from build123d import *

# Parameters (mm, degrees)
SKETCH1_R               = 27.75
SKETCH1_R_2             = 25.75
BOSS_EXTRUDE1_DEPTH     = 2.5
BOSS_EXTRUDE2_START     = -32.750000066
BOSS_EXTRUDE2_OUTLINE_R = 2.5
BOSS_EXTRUDE2_DEPTH     = 65.500000132
BOSS_EXTRUDE2_START_2   = -3
BOSS_EXTRUDE2_2_DEPTH   = 6
CUT_EXTRUDE1_DEPTH      = 43.998546635
CUT_EXTRUDE1_DEPTH_BACK = 43.998546635
SKETCH3_R               = 25.75


with BuildPart() as part:
    # Sketch1 → Boss-Extrude1 (new, symmetric)
    with BuildSketch(Plane(origin=(0, 0, 0), x_dir=(1, 0, 0), z_dir=(0, 1, 0))):
        with Locations(Location((0, 0, 0), (0, 0, 270))):
            Circle(SKETCH1_R)
        with Locations(Location((0, 0, 0), (0, 0, 270))):
            Circle(SKETCH1_R_2, mode=Mode.SUBTRACT)
    extrude(amount=BOSS_EXTRUDE1_DEPTH, both=True)

    # Boss-Extrude2: read off the stored shape, not the designer's step
    # Boss-Extrude2 outline → Boss-Extrude2 (add)
    with BuildSketch(Plane.XY.offset(BOSS_EXTRUDE2_START)):
        Circle(BOSS_EXTRUDE2_OUTLINE_R)
    extrude(amount=BOSS_EXTRUDE2_DEPTH)

    # Boss-Extrude2 2 outline → Boss-Extrude2 2 (cut)
    with BuildSketch(Plane(origin=(0, 0, 0), x_dir=(1, 0, 0), z_dir=(0, 1, 0)).offset(BOSS_EXTRUDE2_START_2)):
        with BuildLine():
            Line((4, -32.539570024), (2.500688791, -32.654387999))
            ThreePointArc((2.500688791, -32.654387999), (1.251258189, -32.726088262), (4.28e-07, -32.75))
            Line((4.28e-07, -32.75), (4, -32.750000066))
            Line((4, -32.750000066), (4, -32.539570024))
        make_face()
        with BuildLine():
            Line((-4, -32.750000066), (4.28e-07, -32.75))
            ThreePointArc((4.28e-07, -32.75), (-1.250913366, -32.726101444), (-2.500001508, -32.654440624))
            Line((-2.500001508, -32.654440624), (-4, -32.539601772))
            Line((-4, -32.539601772), (-4, -32.750000066))
        make_face()
        with BuildLine():
            Line((2.500001316, 32.654440639), (4, 32.539601781))
            Line((4, 32.539601781), (4, 32.750000066))
            Line((4, 32.750000066), (1e-09, 32.75))
            ThreePointArc((1e-09, 32.75), (1.250913484, 32.72610144), (2.500001316, 32.654440639))
        make_face()
        with BuildLine():
            Line((-4, 32.750000066), (-4, 32.539577528))
            Line((-4, 32.539577528), (-2.500526303, 32.654400442))
            ThreePointArc((-2.500526303, 32.654400442), (-1.251176552, 32.726091384), (1e-09, 32.75))
            Line((1e-09, 32.75), (-4, 32.750000066))
        make_face()
    extrude(amount=BOSS_EXTRUDE2_2_DEPTH, mode=Mode.SUBTRACT)

    # Sketch3 → Cut-Extrude1 (cut, two sides: drawn at the far end of the back side and taken through both)
    with BuildSketch(Plane(origin=(0, 0, 0), x_dir=(1, 0, 0), z_dir=(0, 1, 0)).offset(-CUT_EXTRUDE1_DEPTH_BACK)):
        with Locations(Location((0, 0, 0), (0, 0, 270))):
            Circle(SKETCH3_R)
    extrude(amount=CUT_EXTRUDE1_DEPTH + CUT_EXTRUDE1_DEPTH_BACK, mode=Mode.SUBTRACT)


solid = part.part
Build history of the part. All positions in model axes, mm. A direction names the side the tool comes from. Give positions to 0.01 mm unless a question says otherwise; leave off trailing zeros. Write each loop counter-clockwise with the first axis right and the second up, starting at its lowest first coordinate (ties: lowest second). Pieces come first, ordered by that corner, then holes. Notation, with made-up numbers: (-23, -27.75) - (8, -27.75) arc R6 cw to (8, -16.75) - close; hole circle Ø2 at (12, 32.25). An arc over 180 degrees is marked (long way). Use one line per item in the form item = value. Start each with the question number.
1. Band-saw the part on D-D on x = -23.5. Write the cut outline in (y, z), plus the area to 3 significant figures.
2. Two-plate mould, pull along X, no slides. Class faces 3 (the face through (-0.54, -2.44, -30.23)), 4 (the face through (-22.845, -0.035, 11.882)), 5 (the face through (-8, 2.5, 25)): released by +X, released by -X, zero draft, split by the parting line, or undercut.
3. Drop a flat-ended pin along its axis: pin 1 Ø2 at (y, z) = (2, 15) entering from +X. Give the stop position or say it passes through.
4. 3-axis set-ups, long thin cutter, end or side, ignore diameter. For faces 1 (the face through (-8, -2.5, 25)), 2 (the face through (-0.54, -2.44, 30.16)): which of +Z, -Z, +X, -X, +Y, -Y reach the whole face in a straight line?
5. Probe line 1 (X direction, y = -1.35, z = 0); line 2 (Z direction, x = -22, y = -2.1); line 3 (X direction, y = 0.5, z = 18). List the from-to ranges inside material, lowest first. Write a range as [from, to].
6. Band-saw the part on B-B on x = -1.5. Write the cut outline in (y, z), plus the area to 3 significant figures.
7. Band-saw the part on A-A on y = 0. Write the cut outline in (x, z).
8. Band-saw the part on C-C on z = 14.5. Write the cut outline in (x, y).
Conclusion:
q1.outline = (-2.5, -14.76) - (2.5, -14.76) - (2.5, -10.53) - (-2.5, -10.53) - close; (-2.5, 10.53) - (2.5, 10.53) - (2.5, 14.76) - (-2.5, 14.76) - close
q1.area = 42.3 mm²
q2.face_3 = split by the parting line
q2.face_4 = undercut
q2.face_5 = zero draft
q3.pin_1 = 23.96
q4.face_1 = +Z, -Z, +X, -X, -Y
q4.face_2 = +Z
q5.line_1 = [-27.75, -25.75], [25.75, 27.75]
q5.line_2 = [-16.91, -13.38], [13.38, 16.91]
q5.line_3 = [-21.12, -18.41], [18.41, 21.12]
q6.outline = (-2.5, -27.71) - (-2, -27.71) - (-2, -32.72) - (2, -32.72) - (2, -27.71) - (2.5, -27.71) - (2.5, -25.71) - (-2.5, -25.71) - close; (-2.5, 25.71) - (2.5, 25.71) - (2.5, 27.71) - (2, 27.71) - (2, 32.72) - (-2, 32.72) - (-2, 27.71) - (-2.5, 27.71) - close
q6.area = 60.1 mm²
q7.outline = (-2.5, -32.65) arc R32.75 ccw to (2.5, -32.65) - (2.5, -27.64) arc R27.75 ccw to (2.5, 27.64) - (2.5, 32.65) arc R32.75 ccw to (-2.5, 32.65) - (-2.5, 27.64) arc R27.75 ccw to (-2.5, -27.64) - close; hole circle Ø51.5 at (0, 0)
q8.outline = (-23.66, -2.5) - (-21.28, -2.5) - (-21.28, 2.5) - (-23.66, 2.5) - close; (21.28, -2.5) - (23.66, -2.5) - (23.66, 2.5) - (21.28, 2.5) - close
